```python
from build123d import *

# Parameters (mm, degrees)
SKETCH2_W                 = 135
SKETCH2_H                 = 79
BASE_MATERIAL_DEPTH       = 89
THRU_ALL_CUTS_DEPTH       = 136
ANGLE_THRU_ALL_DEPTH      = 21.37861367
ANGLE_THRU_ALL_DEPTH_BACK = 59.62138633
CUT_EXTRUDE3_DEPTH        = 14


with BuildPart() as part:
    # Sketch2 → base-material (new body)
    with BuildSketch(Plane(origin=(0, 0, 0), x_dir=(1, 0, 0), z_dir=(0, 1, 0))):
        with Locations((67.5, 39.5)):
            Rectangle(SKETCH2_W, SKETCH2_H)
    extrude(amount=BASE_MATERIAL_DEPTH)

    # Sketch3 → thru-all-cuts (cut, through all)
    with BuildSketch(Plane(origin=(135, 0, 0), x_dir=(0, 0, -1), z_dir=(1, 0, 0))):
        with BuildLine():
            Line((35.733384694, 89), (79, 89))
            Line((79, 89), (79, 53))
            ThreePointArc((79, 53), (50.857505441, 63.176930949), (35.733384694, 89))
        make_face()
        Polygon((0, 44), (35, 44), (20.37861367, 89), (0, 89), align=None)
    extrude(amount=-THRU_ALL_CUTS_DEPTH, mode=Mode.SUBTRACT)

    # Sketch5 → angle-thru-all (cut, two sides)
    with BuildSketch(Plane.XY.offset(-20.37861367)) as angle_thru_all_sk:
        Polygon((0, 0), (102.382788243, 89), (0, 89), align=None)
    extrude(amount=ANGLE_THRU_ALL_DEPTH, mode=Mode.SUBTRACT)
    extrude(angle_thru_all_sk.sketch, amount=-ANGLE_THRU_ALL_DEPTH_BACK, mode=Mode.SUBTRACT)

    # Sketch7 → Cut-Extrude3 (cut)
    with BuildSketch(Plane.XZ):
        Polygon((27, 0), (52.668656002, -79), (115.756389457, -79), (90.087733454, 0), align=None)
    extrude(amount=-CUT_EXTRUDE3_DEPTH, mode=Mode.SUBTRACT)


solid = part.part
```
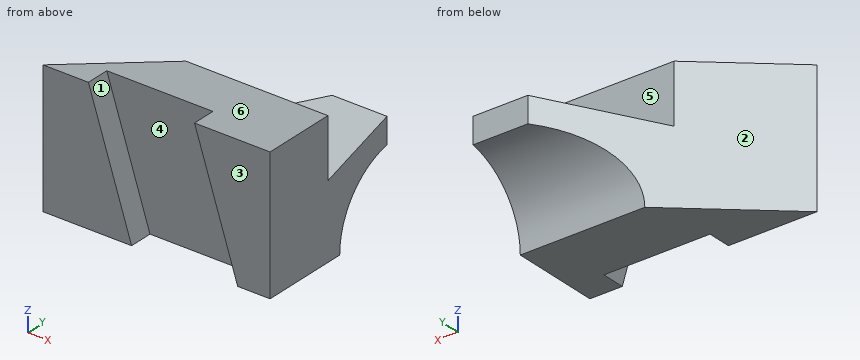
CAD build for the part. Positions are in the model's coordinates, mm. Face numbers are marked on the shaded views. A direction names the side the tool comes from. Coordinates: 2 decimals unless noted, no trailing zeros. Loops run counter-clockwise (first coordinate to the right, second up) from the corner with the lowest first, then second, coordinate; pieces in that order, holes last. Notation, with made-up numbers: (-31, 71) - (12, 71) arc R31 cw to (12, 101) - close; hole circle Ø10 at (-7, 67.5). An arc over 180 degrees is marked (long way). Return JSON: item names as keys, results as strings.
1. Band-saw the part on C-C (x = 104.5). Give the cut face in (y, z).
Result:
{"outline": "(0, -44.36) - (14, -44.36) - (14, -79) - (53, -79) arc R44 cw to (89, -35.73) - (89, -20.38) - (44, -35) - (44, 0) - (0, 0) - close"}
2. 3-axis set-ups, long thin cutter, end or side, ignore diameter. For the marked faces 4, 5 and 6: which of +Z, -Z, +X, -X, +Y, -Y reach the whole face in a straight line?
Result:
{"face 4": "-Y", "face 5": "+Z, +X, -X", "face 6": "+Z, +X, -X, +Y, -Y"}
3. Mould opens along X. For the marked faces 1, 2 and 3 say: released by +X, released by -X, zero draft, split by the parting line, or undercut.
Result:
{"face 1": "undercut", "face 2": "released by -X", "face 3": "zero draft"}
4. Probe L1, parallel to Y at x = 86.5, z = -12; L2, parallel to X at y = 11, z = -37; L3, parallel to Z at x = 92.5, y = 69.5. List the from-to ranges inside material, lowest first. Write a range as from..to.
Result:
{"L1": "y = 14..44", "L2": "x = 12.65..39.02, 102.11..135", "L3": "z = -44.65..-26.71"}
5. Band-saw the part on D-D (z = -11.5). Give the cut face in (x, y), and give its area (3 significant figures).
Result:
{"outline": "(0, 0) - (30.74, 0) - (30.74, 14) - (93.82, 14) - (93.82, 0) - (135, 0) - (135, 44) - (50.62, 44) - close", "area": "3,940 mm2"}
6. Band-saw the part on A-A (z = -24). Give the cut face in (x, y).
Result:
{"outline": "(0, 0) - (34.8, 0) - (34.8, 14) - (97.89, 14) - (97.89, 0) - (135, 0) - (135, 44) - (50.62, 44) - close; (89.56, 77.85) - (135, 77.85) - (135, 89) - (102.38, 89) - close"}
7. Band-saw the part on B-B (y = 8.5). Give the cut face in (x, z).
Result:
{"outline": "(9.78, -79) - (52.67, -79) - (27, 0) - (9.78, 0) - close; (90.09, 0) - (115.76, -79) - (135, -79) - (135, 0) - close"}
8. Drop flat-ended pins along their axis: pin 1 (6 mm diameter, centred on x = 81.5, z = -66.5, fed in from -Y); pin 2 (1.5 mm diameter, centred on x = 69.5, y = 50.5, fed in from +Z); pin 3 (6 mm diameter, centred on y = 10.5, z = -68.5, fed in from -X). Give the stop position or say it passes through.
Result:
{"pin 1": "stops at y = 14", "pin 2": "stops at z = -32.64", "pin 3": "stops at x = 8.63"}
